```python
from build123d import *

# Parameters (mm, degrees)
SKETCH1_W           = 260.096
SKETCH1_H           = 260.096
BOSS_EXTRUDE1_DEPTH = 6.35
SKETCH2_R           = 77.5645
CUT_EXTRUDE1_DEPTH  = 368.886097769
SKETCH3_W           = 12.604
SKETCH3_H           = 50.8
BOSS_EXTRUDE2_DEPTH = 6.35
SKETCH5_R           = 3.175
CUT_EXTRUDE2_DEPTH  = 377.902562629
SKETCH6_R           = 1.5875
CUT_EXTRUDE3_DEPTH  = 377.902562629
SKETCH7_R           = 1.5875
CUT_EXTRUDE4_DEPTH  = 377.902562629
SKETCH8_R           = 0.9525
CUT_EXTRUDE5_DEPTH  = 377.902562629
SKETCH9_R           = 12.7
CUT_EXTRUDE6_DEPTH  = 377.902562629
SKETCH10_R          = 3.175
CUT_EXTRUDE7_DEPTH  = 377.902562629
CAVITY1_START       = 248.539
CAVITY1_OUTLINE_W   = 5.969
CAVITY1_OUTLINE_H   = 6.35
CAVITY1_DEPTH       = 5.207
CAVITY1_START_2     = 240.072333333
CAVITY1_2_OUTLINE_W = 5.207
CAVITY1_2_OUTLINE_H = 6.35
CAVITY1_2_DEPTH     = 4.233333334
SKETCH11_R          = 1.5875
CUT_EXTRUDE8_DEPTH  = 377.902562629


# Read off the part's stored shape, not the designer's step: Cavity1
with BuildPart() as part:
    # Sketch1 → Boss-Extrude1 (new body)
    with BuildSketch(Plane.XY):
        with Locations((130.048, 130.048)):
            Rectangle(SKETCH1_W, SKETCH1_H)
    extrude(amount=BOSS_EXTRUDE1_DEPTH)

    # Sketch2 → Cut-Extrude1 (cut, through all)
    with BuildSketch(Plane.XY.offset(6.35)):
        with Locations((130.048, 130.048)):
            Circle(SKETCH2_R)
    extrude(amount=-CUT_EXTRUDE1_DEPTH, mode=Mode.SUBTRACT)

    # Sketch3 → Boss-Extrude2 (add)
    with BuildSketch(Plane(origin=(0, 0, 0), x_dir=(-1, 0, 0), z_dir=(0, 0, -1))):
        with Locations((-266.398, 234.696)):
            Rectangle(SKETCH3_W, SKETCH3_H)
    extrude(amount=-BOSS_EXTRUDE2_DEPTH)

    # Sketch5 → Cut-Extrude2 (cut, through all)
    with BuildSketch(Plane.XY.offset(6.35)):
        with Locations((193.87464005, 66.22135995)):
            Circle(SKETCH5_R)
        with Locations(Location((66.22135995, 193.87464005, 0), (0, 0, 180))):
            Circle(SKETCH5_R)
        with Locations(Location((193.87464005, 193.87464005, 0), (0, 0, 180))):
            Circle(SKETCH5_R)
        with Locations((66.22135995, 66.22135995)):
            Circle(SKETCH5_R)
    extrude(amount=-CUT_EXTRUDE2_DEPTH, mode=Mode.SUBTRACT)

    # Sketch6 → Cut-Extrude3 (cut, through all)
    with BuildSketch(Plane.XY.offset(6.35)):
        with Locations((264.7625, 253.746)):
            Circle(SKETCH6_R)
        with Locations((264.7625, 215.646)):
            Circle(SKETCH6_R)
        with Locations((204.4375, 253.746)):
            Circle(SKETCH6_R)
        with Locations((204.4375, 215.646)):
            Circle(SKETCH6_R)
    extrude(amount=-CUT_EXTRUDE3_DEPTH, mode=Mode.SUBTRACT)

    # Sketch7 → Cut-Extrude4 (cut, through all)
    with BuildSketch(Plane.XY.offset(6.35)):
        with Locations((248.189, 12.796)):
            Circle(SKETCH7_R)
        with Locations((248.189, 25.496)):
            Circle(SKETCH7_R)
        with Locations((248.189, 38.196)):
            Circle(SKETCH7_R)
        with Locations((84.867, 12.796)):
            Circle(SKETCH7_R)
        with Locations((84.867, 25.496)):
            Circle(SKETCH7_R)
        with Locations((84.867, 38.196)):
            Circle(SKETCH7_R)
        with Locations((12.7, 84.963)):
            Circle(SKETCH7_R)
        with Locations((25.4, 84.963)):
            Circle(SKETCH7_R)
        with Locations((38.1, 84.963)):
            Circle(SKETCH7_R)
        with Locations((38.1, 248.285)):
            Circle(SKETCH7_R)
        with Locations((25.4, 248.285)):
            Circle(SKETCH7_R)
        with Locations((12.7, 248.285)):
            Circle(SKETCH7_R)
    extrude(amount=-CUT_EXTRUDE4_DEPTH, mode=Mode.SUBTRACT)

    # Sketch8 → Cut-Extrude5 (cut, through all)
    with BuildSketch(Plane(origin=(0, 0, 0), x_dir=(-1, 0, 0), z_dir=(0, 0, -1))):
        with Locations((-255.0541, 162.4584)):
            Circle(SKETCH8_R)
        with Locations((-218.0717, 162.4584)):
            Circle(SKETCH8_R)
        with Locations((-166.5986, 218.0717)):
            Circle(SKETCH8_R)
        with Locations((-166.5986, 255.0541)):
            Circle(SKETCH8_R)
        with Locations((-93.4974, 218.0717)):
            Circle(SKETCH8_R)
        with Locations((-93.4974, 255.0541)):
            Circle(SKETCH8_R)
        with Locations((-5.0419, 17.5006)):
            Circle(SKETCH8_R)
        with Locations((-42.0243, 17.5006)):
            Circle(SKETCH8_R)
    extrude(amount=-CUT_EXTRUDE5_DEPTH, mode=Mode.SUBTRACT)

    # Sketch9 → Cut-Extrude6 (cut, through all)
    with BuildSketch(Plane(origin=(0, 0, 0), x_dir=(-1, 0, 0), z_dir=(0, 0, -1))):
        with Locations((-234.6, 234.696)):
            Circle(SKETCH9_R)
    extrude(amount=-CUT_EXTRUDE6_DEPTH, mode=Mode.SUBTRACT)

    # Sketch10 → Cut-Extrude7 (cut, through all)
    with BuildSketch(Plane(origin=(0, 0, 0), x_dir=(-1, 0, 0), z_dir=(0, 0, -1))):
        with Locations((-215.55, 253.746)):
            Circle(SKETCH10_R)
        with Locations((-215.55, 215.646)):
            Circle(SKETCH10_R)
        with Locations((-253.65, 253.746)):
            Circle(SKETCH10_R)
        with Locations((-253.65, 215.646)):
            Circle(SKETCH10_R)
    extrude(amount=-CUT_EXTRUDE7_DEPTH, mode=Mode.SUBTRACT)

    # Cavity1 outline → Cavity1 (cut)
    with BuildSketch(Plane.YZ.offset(CAVITY1_START)):
        with Locations((195.2625, 3.175)):
            Rectangle(CAVITY1_OUTLINE_W, CAVITY1_OUTLINE_H)
    extrude(amount=CAVITY1_DEPTH, mode=Mode.SUBTRACT)

    # Cavity1 2 outline → Cavity1 2 (cut)
    with BuildSketch(Plane.YZ.offset(CAVITY1_START_2)):
        with Locations((201.6125, 3.175)):
            Rectangle(CAVITY1_2_OUTLINE_W, CAVITY1_2_OUTLINE_H)
    extrude(amount=CAVITY1_2_DEPTH, mode=Mode.SUBTRACT)

    # Sketch11 → Cut-Extrude8 (cut, through all)
    with BuildSketch(Plane(origin=(0, 0, 0), x_dir=(-1, 0, 0), z_dir=(0, 0, -1))):
        with Locations((-225.6155, 114.4369)):
            Circle(SKETCH11_R)
        with Locations((-250.8885, 114.4369)):
            Circle(SKETCH11_R)
    extrude(amount=-CUT_EXTRUDE8_DEPTH, mode=Mode.SUBTRACT)


solid = part.part
```
Check sheet for the modelled part. Datum: model origin and axes. Units: mm. A direction names the side the tool comes from. Round coordinates to 2 decimals unless told otherwise and drop trailing zeros. Order: outer loops, then holes, each group sorted by start corner. A loop starts at its lowest first (then second) coordinate and runs counter-clockwise, first axis right, second up. Notation, with made-up numbers: (-36.75, 88.5) - (-28.75, 88.5) arc R17 cw to (-28.75, 94.5) - close; hole circle Ø10 at (-29, 53). An arc over 180 degrees is marked (long way). Answer as CSV lines item,"result". Start each with the question number.
1) Draft check along Y on faces 4 (the face through (266, 209.296, 3)), 5 (the face through (255.99, 217.79, 3.13)), 6 (the face through (199, 190, 0)). Enter one of: +Y half, -Y half, draft (parallel to the pull), parting line (faces both ways), or undercut.
2) Tool access check on faces 1 (the face through (0, 128, 3)), 2 (the face through (248.539, 195, 3)), 3 (the face through (260.096, 103, 3)). Record the directions out of +Z, -Z, +X, -X, +Y, -Y that give a thin tool (end or side, any length) a straight path to the whole face; none if there is none.
3) Section check A-A (y = 231). Record the cut outline in (x, z), then the cut area to 3 significant figures.
4) Section check B-B (x = 180). Record the cut outline in (y, z), then the cut area to 3 significant figures.
5) Depth check by flat-ended pin: pin 1 (1.1 mm diameter, centred on x = 218.07, y = 162.46, fed in from -Z); pin 2 (3 mm diameter, centred on y = 112, z = 3, fed in from +X). Enter the tip coordinate at first touch or a pass-through.
6) Scan lines: probe 1 along Y at (x, z) = (253.65, 4.75); probe 2 along X at (y, z) = (248, 3); probe 3 along Y at (x, z) = (25, 5.75). Record each from-to range of solid material in increasing order.
7) Section check C-C (z = 5). Give the number of separate pieces and of enclosed holes in the cut face, then the cut area to 3 significant figures.
Determined:
1,face 4,"-Y half"
1,face 5,"undercut"
1,face 6,"draft"
2,face 1,"+Z, -Z, -X, +Y, -Y"
2,face 2,"+Z, -Z"
2,face 3,"+Z, -Z, +X, -Y"
3,outline,"(0, 0) - (222.45, 0) - (222.45, 6.35) - (0, 6.35) - close; (246.75, 0) - (272.7, 0) - (272.7, 6.35) - (246.75, 6.35) - close"
3,area,"1,580 mm^2"
4,outline,"(0, 0) - (70.71, 0) - (70.71, 6.35) - (0, 6.35) - close; (189.39, 0) - (260.1, 0) - (260.1, 6.35) - (189.39, 6.35) - close"
4,area,"898 mm^2"
5,pin 1,"through"
5,pin 2,"x = 260.1"
6,probe 1,"0 to 192.28, 198.25 to 212.47, 218.82 to 250.57, 256.92 to 260.1"
6,probe 2,"0 to 11.14, 14.26 to 23.84, 26.96 to 36.54, 39.66 to 272.7"
6,probe 3,"0 to 83.43, 86.5 to 246.75, 249.82 to 260.1"
7,separate pieces,"1"
7,enclosed holes,"38"
7,area,"48,400 mm^2"
